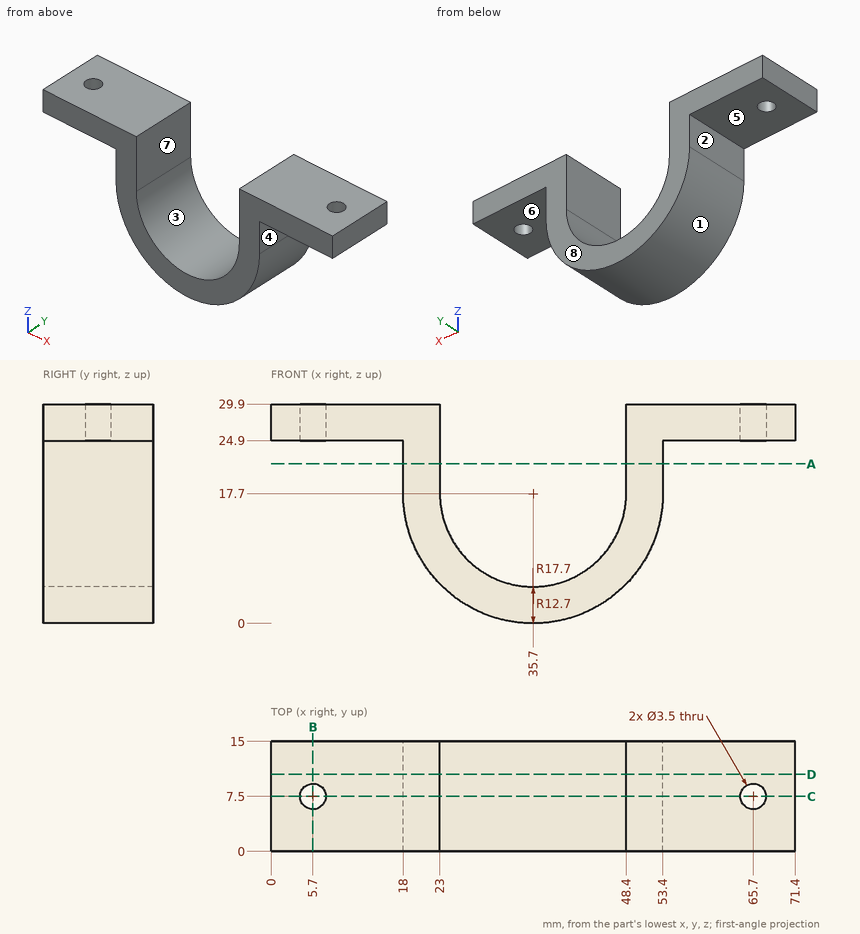
Input: dimensioned drawing with shaded views. Units: mm. Origin: part minimum x, y, z. A direction names the side the tool comes from. Round coordinates to 2 decimals unless told otherwise and drop trailing zeros. Order: outer loops, then holes, each group sorted by start corner. A loop starts at its lowest first (then second) coordinate and runs counter-clockwise, first axis right, second up. Notation, with made-up numbers: (-23.5, 20) - (-8.5, 20) arc R14 cw to (-8.5, 45) - close; hole circle Ø1 at (-30.5, 75). An arc over 180 degrees is marked (long way). Answer as a JSON object with one key per item and string values. Group by question number.
(1) Cut plane B-B (x = 5.7). Return loops of the section in (y, z), then the cut area to 3 significant figures.
(2) Material intervals for probe 1 along Y at (x, z) = (65.7, 28.25); probe 2 along X at (y, z) = (0.75, 21.75); probe 3 along Z at (x, y) = (58.5, 10.25), sorted ascending. Write a range as from..to.
(3) Cut plane D-D (y = 10.5). Return loops of the section in (x, z).
(4) Draft query along X for the marked faces 1, 2, 3 and 4. Return one class per face: released by +X, released by -X, zero draft, split by the parting line, or undercut.
(5) Reachability of the marked faces 5, 6, 7 and 8 from +Z, -Z, +X, -X, +Y, -Y: full face, straight path, thin tool, end or side. Return the list, or none.
(6) Cut plane A-A (z = 21.75). Return loops of the section in (x, y).
(7) Cut plane C-C (y = 7.5). Return loops of the section in (x, z).
(8) Pin query (flat end, axial travel): P1, Ø8, axis at y = 4, z = 15.5, coming from the +X side; P2, Ø3, axis at y = 2, z = 9, coming from the +X side; P3, Ø1.5, axis at x = 44, y = 7, coming from the +Z side. Return the tip coordinate at first contact, or that it passes through.
Here are the results:
{
 "1": {"outline": "(0, 24.9) - (5.75, 24.9) - (5.75, 29.9) - (0, 29.9) - close; (9.25, 24.9) - (15, 24.9) - (15, 29.9) - (9.25, 29.9) - close", "area": "57.5 mm^2"},
 "2": {"probe 1": "y = 0..5.75, 9.25..15", "probe 2": "x = 18..23, 48.4..53.4", "probe 3": "z = 24.9..29.9"},
 "3": {"outline": "(0, 24.9) - (18, 24.9) - (18, 17.7) arc R17.7 ccw to (53.4, 17.7) - (53.4, 24.9) - (71.4, 24.9) - (71.4, 29.9) - (48.4, 29.9) - (48.4, 17.7) arc R12.7 cw to (23, 17.7) - (23, 29.9) - (0, 29.9) - close"},
 "4": {"face 1": "split by the parting line", "face 2": "released by -X", "face 3": "undercut", "face 4": "released by +X"},
 "5": {"face 5": "-Z, -X, +Y, -Y", "face 6": "-Z, +X, +Y, -Y", "face 7": "+Z, +Y, -Y", "face 8": "+Z, -Z, +X, -X, +Y"},
 "6": {"outline": "(18, 0) - (23, 0) - (23, 15) - (18, 15) - close; (48.4, 0) - (53.4, 0) - (53.4, 15) - (48.4, 15) - close"},
 "7": {"outline": "(0, 24.9) - (3.95, 24.9) - (3.95, 29.9) - (0, 29.9) - close; (7.45, 24.9) - (18, 24.9) - (18, 17.7) arc R17.7 ccw to (53.4, 17.7) - (53.4, 24.9) - (63.95, 24.9) - (63.95, 29.9) - (48.4, 29.9) - (48.4, 17.7) arc R12.7 cw to (23, 17.7) - (23, 29.9) - (7.45, 29.9) - close; (67.45, 24.9) - (71.4, 24.9) - (71.4, 29.9) - (67.45, 29.9) - close"},
 "8": {"P1": "stops at x = 53.4", "P2": "stops at x = 51.87", "P3": "stops at z = 8.79"}
}
